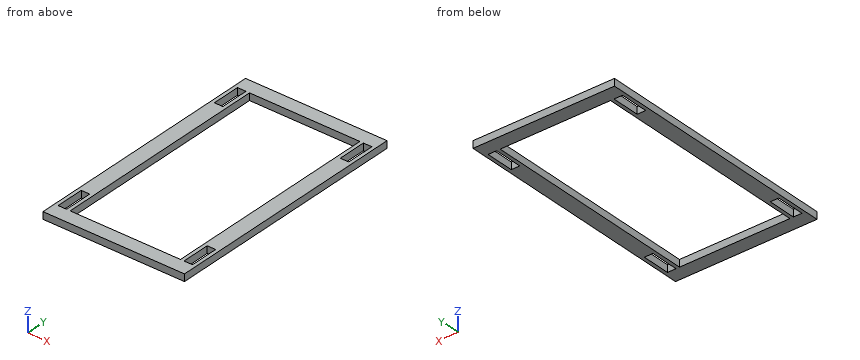
```python
from build123d import *

# Parameters (mm, degrees)
F0_W     = 100
F0_H     = 175
F0_W_2   = 6
F0_H_2   = 20
F0_W_3   = 78
F0_H_3   = 155
F1_DEPTH = 5


with BuildPart() as f1:
    # F0 (on Top) → F1 (new body)
    with BuildSketch(Plane.XY):
        Rectangle(F0_W, F0_H)
        with Locations((-44.5, -67.5)):
            Rectangle(F0_W_2, F0_H_2, mode=Mode.SUBTRACT)
        with Locations((44.5, -67.5)):
            Rectangle(F0_W_2, F0_H_2, mode=Mode.SUBTRACT)
        with Locations((-44.5, 67.5)):
            Rectangle(F0_W_2, F0_H_2, mode=Mode.SUBTRACT)
        Rectangle(F0_W_3, F0_H_3, mode=Mode.SUBTRACT)
        with Locations((44.5, 67.5)):
            Rectangle(F0_W_2, F0_H_2, mode=Mode.SUBTRACT)
    extrude(amount=F1_DEPTH)


solid = f1.part
```
Can you work these out from the model? Positions are in its coordinate system, mm. Round coordinates to 2 decimals unless told otherwise and drop trailing zeros. Order: outer loops, then holes, each group sorted by start corner. A loop starts at its lowest first (then second) coordinate and runs counter-clockwise, first axis right, second up.
(1) If we section it at D-D (z = 1.5): Please give me the cut outline in (x, y), plus the area to 3 significant figures.
Results are:
outline: (-50, -87.5) - (50, -87.5) - (50, 87.5) - (-50, 87.5) - close; hole (-47.5, -77.5) - (-41.5, -77.5) - (-41.5, -57.5) - (-47.5, -57.5) - close; hole (-47.5, 57.5) - (-41.5, 57.5) - (-41.5, 77.5) - (-47.5, 77.5) - close; hole (-39, -77.5) - (39, -77.5) - (39, 77.5) - (-39, 77.5) - close; hole (41.5, -77.5) - (47.5, -77.5) - (47.5, -57.5) - (41.5, -57.5) - close; hole (41.5, 57.5) - (47.5, 57.5) - (47.5, 77.5) - (41.5, 77.5) - close
area: 4,930 mm2
(2) If we section it at B-B (y = -68.5): Please give me the cut outline in (x, z), plus the area to 3 significant figures.
Results are:
outline: (-50, 0) - (-47.5, 0) - (-47.5, 5) - (-50, 5) - close; (-41.5, 0) - (-39, 0) - (-39, 5) - (-41.5, 5) - close; (39, 0) - (41.5, 0) - (41.5, 5) - (39, 5) - close; (47.5, 0) - (50, 0) - (50, 5) - (47.5, 5) - close
area: 50.0 mm2
(3) If we section it at A-A (y = -25): Please give me the cut outline in (x, z), plus the area to 3 significant figures.
Results are:
outline: (-50, 0) - (-39, 0) - (-39, 5) - (-50, 5) - close; (39, 0) - (50, 0) - (50, 5) - (39, 5) - close
area: 110 mm2
(4) If I drill on L1, parallel to X at y = 69.5, z = 3.6; L2, parallel to Y at x = -43, z = 3.55; L3, parallel to X at y = -25, z = 2.6, over which ranges is the centre line in solid material (lowest first)?
Results are:
L1: x = -50 to -47.5, -41.5 to -39, 39 to 41.5, 47.5 to 50
L2: y = -87.5 to -77.5, -57.5 to 57.5, 77.5 to 87.5
L3: x = -50 to -39, 39 to 50
(5) If we section it at C-C (x = 27.5): Please give me the cut outline in (y, z), plus the area to 3 significant figures.
Results are:
outline: (-87.5, 0) - (-77.5, 0) - (-77.5, 5) - (-87.5, 5) - close; (77.5, 0) - (87.5, 0) - (87.5, 5) - (77.5, 5) - close
area: 100 mm2
